from build123d import *

# Parameters (mm, degrees)
SKETCH_1_W               = 60
SKETCH_1_H               = 44
SKETCH_1_R               = 1.6
EXTRUDE_1_DEPTH          = 1
SKETCH_2_W               = 134.5
SKETCH_2_H               = 90
EXTRUDE_2_DEPTH          = 1
CUT_EXTRUDE_1_DEPTH      = 2
SKETCH_4_R               = 1.6
CUT_EXTRUDE_2_DEPTH      = 2
SKETCH_5_R               = 1.35
CUT_EXTRUDE_3_DEPTH      = 2
SKETCH_6_W               = 15
SKETCH_6_H               = 90
CUT_EXTRUDE_4_DEPTH      = 1
CUT_EXTRUDE_4_DEPTH_BACK = 2
SKETCH_7_W               = 9
SKETCH_7_H               = 22.5
CUT_EXTRUDE_5_DEPTH      = 2
FILLET_1_R               = 2
CUT_EXTRUDE_6_DEPTH      = 2
CUT_EXTRUDE_7_DEPTH      = 2
CHAMFER_2_SIZE           = 3
CHAMFER_2_EDGE_2_SIZE    = 3
CHAMFER_2_EDGE_3_SIZE2   = 3
CHAMFER_2_EDGE_3_SIZE    = 2.449489743
CHAMFER_2_EDGE_4_SIZE2   = 4.242640687
CHAMFER_2_EDGE_4_SIZE    = 3


with BuildPart() as part:
    # 草图1 → 凸台-拉伸1 (new body)
    with BuildSketch(Plane(origin=(0, 0, 0), x_dir=(0, 0, -1), z_dir=(1, 0, 0))):
        with Locations((18, -14.5)):
            Rectangle(SKETCH_1_W, SKETCH_1_H)
        Circle(SKETCH_1_R, mode=Mode.SUBTRACT)
        with Locations((17, 0)):
            Circle(SKETCH_1_R, mode=Mode.SUBTRACT)
        with Locations((0, -30.5)):
            Circle(SKETCH_1_R, mode=Mode.SUBTRACT)
        with Locations((17, -30.5)):
            Circle(SKETCH_1_R, mode=Mode.SUBTRACT)
        with Locations((31.5, -30.5)):
            Circle(SKETCH_1_R, mode=Mode.SUBTRACT)
    extrude(amount=EXTRUDE_1_DEPTH)

    # 草图2 → 凸台-拉伸2 (add)
    with BuildSketch(Plane(origin=(1, 0, 0), x_dir=(0, 0, -1), z_dir=(1, 0, 0))):
        with Locations((-19.25, 52.5)):
            Rectangle(SKETCH_2_W, SKETCH_2_H)
    extrude(amount=-EXTRUDE_2_DEPTH)

    # 草图3 → 切除-拉伸1 (cut, through all)
    with BuildSketch(Plane.ZY):
        Polygon((86.5, 7.5), (62.384572681, 97.5), (86.5, 97.5), align=None)
    extrude(amount=-CUT_EXTRUDE_1_DEPTH, mode=Mode.SUBTRACT)

    # 草图4 → 切除-拉伸2 (cut, through all)
    with BuildSketch(Plane.ZY):
        with Locations((71.5, 10.5)):
            Circle(SKETCH_4_R)
        with Locations((51.5, 10.5)):
            Circle(SKETCH_4_R)
        with Locations((12, 94.5)):
            Circle(SKETCH_4_R)
        with Locations((32, 94.5)):
            Circle(SKETCH_4_R)
        with Locations((65.977473951, 72.5)):
            Circle(SKETCH_4_R)
        with Locations((76.330235755, 33.862966948)):
            Circle(SKETCH_4_R)
    extrude(amount=-CUT_EXTRUDE_2_DEPTH, mode=Mode.SUBTRACT)

    # 草图5 → 切除-拉伸3 (cut, through all)
    with BuildSketch(Plane(origin=(1, 0, 0), x_dir=(0, 0, -1), z_dir=(1, 0, 0))):
        with Locations((-26.5, 55.5)):
            Circle(SKETCH_5_R)
        with Locations((9.5, 55.5)):
            Circle(SKETCH_5_R)
        with Locations((9.5, 19.5)):
            Circle(SKETCH_5_R)
        with Locations((-26.5, 19.5)):
            Circle(SKETCH_5_R)
    extrude(amount=-CUT_EXTRUDE_3_DEPTH, mode=Mode.SUBTRACT)

    # 草图6 → 切除-拉伸4 (cut, two sides)
    with BuildSketch(Plane(origin=(1, 0, 0), x_dir=(0, 0, -1), z_dir=(1, 0, 0))) as cut_extrude_4_sk:
        with Locations((40.5, 52.5)):
            Rectangle(SKETCH_6_W, SKETCH_6_H)
    extrude(amount=CUT_EXTRUDE_4_DEPTH, mode=Mode.SUBTRACT)
    extrude(cut_extrude_4_sk.sketch, amount=-CUT_EXTRUDE_4_DEPTH_BACK, mode=Mode.SUBTRACT)

    # 草图7 → 切除-拉伸5 (cut, through all)
    with BuildSketch(Plane(origin=(1, 0, 0), x_dir=(0, 0, -1), z_dir=(1, 0, 0))):
        with Locations((8.5, -15.25)):
            Rectangle(SKETCH_7_W, SKETCH_7_H)
    extrude(amount=-CUT_EXTRUDE_5_DEPTH, mode=Mode.SUBTRACT)

    # 圆角1
    fillet_1_edges = [part.edges().sort_by_distance(p)[0] for p in [
        (0.5, -4, -13),
        (0.5, -26.5, -13),
        (0.5, -26.5, -4),
        (0.5, -4, -4),
    ]]
    fillet(fillet_1_edges, radius=FILLET_1_R)

    # 草图8 → 切除-拉伸6 (cut, through all)
    with BuildSketch(Plane(origin=(1, 0, 0), x_dir=(0, 0, -1), z_dir=(1, 0, 0))):
        Polygon((-12, 7.5), (33, 7.5), (48, 7.5), (48, -36.5), (-12, -36.5), align=None)
    extrude(amount=-CUT_EXTRUDE_6_DEPTH, mode=Mode.SUBTRACT)

    # 草图9 → 切除-拉伸7 (cut, through all)
    with BuildSketch(Plane(origin=(1, 0, 0), x_dir=(0, 0, -1), z_dir=(1, 0, 0))):
        with BuildLine():
            Line((-18.5, 63.5), (1.5, 63.5))
            ThreePointArc((1.5, 63.5), (3, 62), (1.5, 60.5))
            Line((1.5, 60.5), (-18.5, 60.5))
            ThreePointArc((-18.5, 60.5), (-20, 62), (-18.5, 63.5))
        make_face()
        with BuildLine():
            Line((-32.5, 47.5), (-32.5, 27.5))
            ThreePointArc((-32.5, 27.5), (-34, 26), (-35.5, 27.5))
            Line((-35.5, 27.5), (-35.5, 47.5))
            ThreePointArc((-35.5, 47.5), (-34, 49), (-32.5, 47.5))
        make_face()
        with BuildLine():
            Line((15.5, 47.5), (15.5, 27.5))
            ThreePointArc((15.5, 27.5), (17, 26), (18.5, 27.5))
            Line((18.5, 27.5), (18.5, 47.5))
            ThreePointArc((18.5, 47.5), (17, 49), (15.5, 47.5))
        make_face()
    extrude(amount=-CUT_EXTRUDE_7_DEPTH, mode=Mode.SUBTRACT)

    # 倒角2
    chamfer_2_edges = [part.edges().sort_by_distance(p)[0] for p in [
        (0.5, 7.5, -33),
    ]]
    chamfer(chamfer_2_edges, length=CHAMFER_2_SIZE)

    # 倒角2 edge 2
    chamfer_2_edge_2_edges = [part.edges().sort_by_distance(p)[0] for p in [
        (0.5, 97.5, -33),
    ]]
    chamfer(chamfer_2_edge_2_edges, length=CHAMFER_2_EDGE_2_SIZE)

    # 倒角2 edge 3
    chamfer_2_edge_3_edges = [part.edges().sort_by_distance(p)[0] for p in [
        (0.5, 7.5, 86.5),
    ]]
    chamfer(chamfer_2_edge_3_edges, length=CHAMFER_2_EDGE_3_SIZE, length2=CHAMFER_2_EDGE_3_SIZE2)

    # 倒角2 edge 4
    chamfer_2_edge_4_edges = [part.edges().sort_by_distance(p)[0] for p in [
        (0.5, 97.5, 62.384572681),
    ]]
    chamfer(chamfer_2_edge_4_edges, length=CHAMFER_2_EDGE_4_SIZE, length2=CHAMFER_2_EDGE_4_SIZE2)


solid = part.part
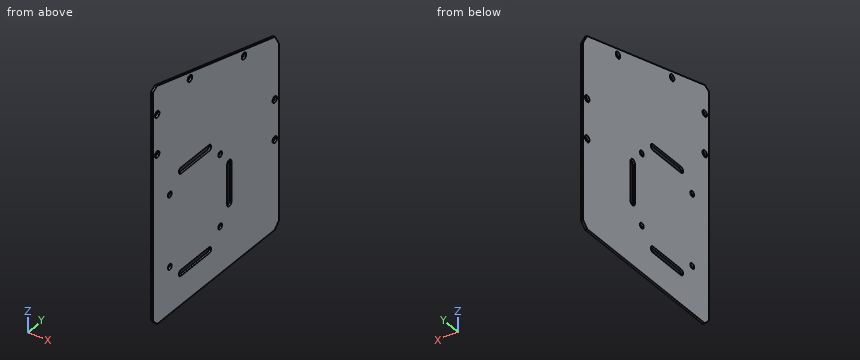
The listing builds one solid part. Answer for the finished solid, in the listing's coordinates (mm). Coordinates: 2 decimals unless noted, no trailing zeros. Loops run counter-clockwise (first coordinate to the right, second up) from the corner with the lowest first, then second, coordinate; pieces in that order, holes last.
1) Find section A-A on z = 51.5. Write down the section's boundary in (x, y), then the cut area to 3 significant figures.
2) Find section D-D on x = 0.3. Give the number of separate pieces and of enclosed holes in the cut face, then the cut area to 3 significant figures.
3) Find section C-C on z = -9.5. Write down the section's boundary in (x, y), then the cut area to 3 significant figures.
4) Find section B-B on y = 19.5. Write down the section's boundary in (x, z), then the cut area to 3 significant figures.
5) Find the intervals of material crossed by L1, parallel to Y at x = 0.6, z = -9.5; L2, parallel to Z at x = 0.8, y = 94.5; L3, parallel to Y at x = 0.2, z = 12, in increasing order.
6) Flat-ended cylindrical pins translate along their axes: pin 1 Ø2.5 at (y, z) = (10.5, 51.5) entering from +X; pin 2 Ø0.5 at (x, y) = (0.5, 35) entering from +Z. Find the tip coordinate at first contact, or state that the pin passes through.
Values:
1. outline: (0, 7.5) - (1, 7.5) - (1, 8.9) - (0, 8.9) - close; (0, 12.1) - (1, 12.1) - (1, 97.5) - (0, 97.5) - close
1. area: 86.8 mm2
2. separate pieces: 1
2. enclosed holes: 13
2. area: 9,380 mm2
3. outline: (0, 7.5) - (1, 7.5) - (1, 18.15) - (0, 18.15) - close; (0, 20.85) - (1, 20.85) - (1, 54.15) - (0, 54.15) - close; (0, 56.85) - (1, 56.85) - (1, 97.5) - (0, 97.5) - close
3. area: 84.6 mm2
4. outline: (0, -33) - (1, -33) - (1, -10.85) - (0, -10.85) - close; (0, -8.15) - (1, -8.15) - (1, 25.15) - (0, 25.15) - close; (0, 27.85) - (1, 27.85) - (1, 83.28) - (0, 83.28) - close
4. area: 111 mm2
5. L1: y = 7.5 to 18.15, 20.85 to 54.15, 56.85 to 97.5
5. L2: z = -33 to 10.4, 13.6 to 30.4, 33.6 to 63.19
5. L3: y = 7.5 to 60.5, 63.5 to 92.9, 96.1 to 97.5
6. pin 1: passes through
6. pin 2: stops at z = 79.2
